CAD build for the part. Positions are in the model's coordinates, mm. Give positions to 0.01 mm unless a question says otherwise; leave off trailing zeros. Loops run counter-clockwise (first coordinate to the right, second up) from the corner with the lowest first, then second, coordinate; pieces in that order, holes last.
Item 1: Saw through at A-A on y = 6.35. Give the cut face in (x, z) (3 decimals).
Item 2: Drop a flat-ended pin along its axis: P1, Ø4, axis at x = 6.5, y = 15.5, coming from the -Z side. Give the stop position or say it passes through.
Item 3: Saw through at D-D on y = 19.05. Give the cut face in (x, z) (3 decimals), plus the area to 3 significant figures.
Item 4: Probe probe 1 along Y at (x, z) = (48.55, 19.05); probe 2 along X at (y, z) = (8.25, 8.75) (3 decimals); probe 3 along Y at (x, z) = (19, 1.75) (3 decimals). List the from-to ranges inside material, lowest first.
Item 5: Saw through at B-B on z = 1.5. Give the cut face in (x, y) (3 decimals).
Item 6: Saw through at C-C on y = 14.75. Give the cut face in (x, z) (3 decimals), plus the area to 3 significant figures.
Item 7: Mould opens along Z. For faces 1 (the flat face through (7, 24, 3.175)), 2 (the cylindrical face through (10.276, 1.565, 3.871)) say: released by +Z, released by -Z, zero draft, split by the parting line, or undercut.
Autodesk Inventor part; units mm, degrees
ref_plane "YZ Plane" through (0, 0, 0) normal (1, 0, 0) x (0, 1, 0)
ref_plane "XZ Plane" through (0, 0, 0) normal (0, 1, 0) x (-1, 0, 0)
ref_plane "XY Plane" through (0, 0, 0) normal (0, 0, 1) x (1, 0, 0)
sketch "Sketch1" plane through (0, 0, 0) normal (0, 0, 1) x (1, 0, 0)
  line L0 (0, 0) -> (50.8, 0)
  line L1 (50.8, 0) -> (50.8, 25.4)
  line L2 (50.8, 25.4) -> (0, 25.4)
  line L3 (0, 25.4) -> (0, 0)
  line L4 (3.175, 22.225) -> (47.625, 22.225)
  line L5 (47.625, 22.225) -> (47.625, 3.175)
  line L6 (47.625, 3.175) -> (3.175, 3.175)
  line L7 (3.175, 3.175) -> (3.175, 22.225)
  dimension "d0" = 50.8
  dimension "d1" = 25.4
  dimension "d2" = 3.175
  dimension "d3" = 3.175
  dimension "d4" = 3.175
  dimension "d5" = 3.175
extrude "Extrusion1" add sketch "Sketch1" along normal blind 25.4
sketch "Sketch2" plane through (0, 25.4, 0) normal (0, 1, 0) x (1, 0, 0)
  line L0 (0, -25.4) -> (50.8, -25.4)
  line L1 (50.8, 0) -> (50.8, -25.4)
  line L2 (0, 0) -> (0, -25.4)
  line L3 (3.175, -22.225) -> (3.175, -3.175)
  line L4 (47.625, -22.225) -> (3.175, -22.225)
  line L5 (3.175, -3.175) -> (47.625, -3.175)
  line L6 (27.7711, -3.175) -> (21.3007, -18.2093)
  line L7 (29.4993, -3.175) -> (21.3007, -22.225) construction
  line L8 (29.4993, -7.1907) -> (23.0289, -22.225)
  line L9 (35.9698, -22.225) -> (29.4993, -7.1907)
  line L10 (37.698, -22.225) -> (29.4993, -3.175) construction
  line L11 (37.698, -18.2093) -> (31.2276, -3.175)
  line L12 (44.1684, -3.175) -> (37.698, -18.2093)
  line L13 (45.8967, -3.175) -> (37.698, -22.225) construction
  line L14 (39.4263, -22.225) -> (47.625, -3.175)
  line L15 (47.625, -3.175) -> (47.625, -22.225)
  line L16 (21.3007, -18.2093) -> (14.8302, -3.175)
  line L17 (21.3007, -22.225) -> (13.102, -3.175) construction
  line L18 (19.5724, -22.225) -> (13.102, -7.1907)
  line L19 (13.102, -7.1907) -> (6.6316, -22.225)
  line L20 (13.102, -3.175) -> (4.9033, -22.225) construction
  line L21 (3.175, -22.225) -> (11.3737, -3.175)
  line L22 (50.8, 0) -> (0, 0)
  dimension "d9" = 1.5875
  dimension "d10" = 3.175
  dimension "d11" = 1.5875
  dimension "d12" = 3.175
  dimension "d13" = 1.5875
  dimension "d14" = 3.175
  dimension "d15" = 1.5875
  dimension "d16" = 3.175
  dimension "d17" = 1.5875
  dimension "d18" = 3.175
  dimension "d19" = 23.286
  dimension "d20" = 46.572
  dimension "d21" = 46.572
  dimension "d22" = 46.572
  dimension "d23" = 46.572
  dimension "d24" = 3.175
  dimension "d26" = 3.175
  dimension "d27" = 3.175
  dimension "d32" = 3.175
extrude "Extrusion2" cut sketch "Sketch2" against normal blind 76.2 contours L3 L5 L21 | L19 L18 L4 | L5 L6 L16 | L8 L9 L4 | L5 L12 L11 | L14 L15 L4
fillet "Fillet1" radius 1.5875 18 edges at (3.175, 23.8125, 3.175) (11.3737, 23.8125, 3.175) (3.175, 23.8125, 22.225) (13.102, 23.8125, 7.1907) (6.6316, 23.8125, 22.225) (19.5724, 23.8125, 22.225) (14.8302, 23.8125, 3.175) (21.3007, 23.8125, 18.2093) (27.7711, 23.8125, 3.175) (29.4993, 23.8125, 7.1907) (23.0289, 23.8125, 22.225) (35.9698, 23.8125, 22.225) (31.2276, 23.8125, 3.175) (37.698, 23.8125, 18.2093) (44.1684, 23.8125, 3.175) (47.625, 23.8125, 3.175) (39.4263, 23.8125, 22.225) (47.625, 23.8125, 22.225)
fillet "Fillet2" radius 1.5875 18 edges at (11.3737, 1.5875, 3.175) (3.175, 1.5875, 3.175) (3.175, 1.5875, 22.225) (6.6316, 1.5875, 22.225) (13.102, 1.5875, 7.1907) (19.5724, 1.5875, 22.225) (21.3007, 1.5875, 18.2093) (14.8302, 1.5875, 3.175) (27.7711, 1.5875, 3.175) (29.4993, 1.5875, 7.1907) (23.0289, 1.5875, 22.225) (35.9698, 1.5875, 22.225) (37.698, 1.5875, 18.2093) (31.2276, 1.5875, 3.175) (44.1684, 1.5875, 3.175) (47.625, 1.5875, 3.175) (39.4263, 1.5875, 22.225) (47.625, 1.5875, 22.225)
sketch "Sketch3" plane through (50.8, 0, 0) normal (1, 0, 0) x (0, 0, -1)
  line L0 (-25.4, 25.4) -> (-25.4, 0)
  line L1 (0, 0) -> (-25.4, 0)
  line L2 (0, 0) -> (0, 25.4)
  line L3 (0, 25.4) -> (-25.4, 25.4)
  circle A0 centre (-19.05, 19.05) radius 1.7272
  circle A1 centre (-19.05, 6.35) radius 1.7272
  circle A2 centre (-6.35, 19.05) radius 1.7272
  dimension "d33" = 3.4544
  dimension "d34" = 6.35
  dimension "d35" = 6.35
  dimension "d36" = 6.35
  dimension "d37" = 6.35
extrude "Extrusion3" cut sketch "Sketch3" against normal through all contours A0 | A1 | A2
equation "\"d3\" = d2"
equation "\"d4\" = d2"
equation "\"d5\" = d2"
equation "\"d10\" = 2 * d9"
equation "\"d11\" = d9"
equation "\"d12\" = d10"
equation "\"d13\" = d11"
equation "\"d15\" = d13"
equation "\"d16\" = d14"
equation "\"d17\" = d15"
equation "\"d18\" = d16"
equation "\"d20\" = 2 * d19"
equation "\"d21\" = d20"
equation "\"d22\" = d21"
equation "\"d23\" = d22"
equation "\"d36\" = d35"
equation "\"d37\" = d34"
properties part number "1x2 Aluminum Tube Corner Post"
Results below:
1. outline: (0, 0) - (3.175, 0) - (3.175, 17.323) - (0, 17.323) - close; (0, 20.777) - (3.175, 20.777) - (3.175, 25.4) - (0, 25.4) - close; (47.625, 0) - (50.8, 0) - (50.8, 17.323) - (47.625, 17.323) - close; (47.625, 20.777) - (50.8, 20.777) - (50.8, 25.4) - (47.625, 25.4) - close
2. P1: passes through
3. outline: (0, 0) - (3.175, 0) - (3.175, 4.623) - (0, 4.623) - close; (0, 8.077) - (3.175, 8.077) - (3.175, 17.323) - (0, 17.323) - close; (0, 20.777) - (3.175, 20.777) - (3.175, 25.4) - (0, 25.4) - close; (47.625, 0) - (50.8, 0) - (50.8, 4.623) - (47.625, 4.623) - close; (47.625, 8.077) - (50.8, 8.077) - (50.8, 17.323) - (47.625, 17.323) - close; (47.625, 20.777) - (50.8, 20.777) - (50.8, 25.4) - (47.625, 25.4) - close
3. area: 117 mm2
4. probe 1: y = 0 to 4.62, 8.08 to 17.32, 20.78 to 25.4
4. probe 2: x = 0 to 3.175, 47.625 to 50.8
4. probe 3: y = 0 to 3.175, 22.225 to 25.4
5. outline: (0, 0) - (50.8, 0) - (50.8, 25.4) - (0, 25.4) - close; hole (3.175, 3.175) - (47.625, 3.175) - (47.625, 22.225) - (3.175, 22.225) - close
6. outline: (0, 0) - (3.175, 0) - (3.175, 25.4) - (0, 25.4) - close; (47.625, 0) - (50.8, 0) - (50.8, 25.4) - (47.625, 25.4) - close
6. area: 161 mm2
7. face 1: undercut
7. face 2: undercut
